Here's how the part is built. I have some questions about the finished solid (model axes, mm). Face numbers are marked on the shaded views. A direction names the side the tool comes from. Coordinates: 2 decimals unless noted, no trailing zeros. Write each loop counter-clockwise with the first axis right and the second up, starting at its lowest first coordinate (ties: lowest second). Pieces come first, ordered by that corner, then holes.
from build123d import *

# Parameters (mm, degrees)
F0_W     = 54
F0_H     = 150
F1_DEPTH = 50
F2_R     = 15
F3_R     = 15
F5_DEPTH = 5
F6_W     = 121.107407
F6_H     = 220.926333
F7_DEPTH = 5.001
F8_W     = 141.400545
F8_H     = 89.871116
F9_DEPTH = 50.001
F10_T    = -2.5


with BuildPart() as f1:
    # F0 (on Top) → F1 (new body)
    with BuildSketch(Plane.XY):
        Rectangle(F0_W, F0_H)
    extrude(amount=F1_DEPTH)

    # F2
    f2_edges = [f1.edges().sort_by_distance(p)[0] for p in [
        (27, -75, 25),
        (-27, -75, 25),
        (27, 75, 25),
        (-27, 75, 25),
    ]]
    fillet(f2_edges, radius=F2_R)

    # F3
    f3_edges = [f1.edges().sort_by_distance(p)[0] for p in [
        (-27, 0, 50),
    ]]
    fillet(f3_edges, radius=F3_R)

    # F4 (on face) → F5 (join)
    with BuildSketch(Plane(origin=(0, 0, 0), x_dir=(1, 0, 0), z_dir=(0, 0, -1))):
        with BuildLine():
            ThreePointArc((12, -75), (22.606602, -70.606602), (27, -60))
            Line((27, -60), (27, 60))
            ThreePointArc((27, 60), (22.606602, 70.606602), (12, 75))
            Line((12, 75), (-12, 75))
            ThreePointArc((-12, 75), (-22.606602, 70.606602), (-27, 60))
            Line((-27, 60), (-27, -60))
            ThreePointArc((-27, -60), (-22.606602, -70.606602), (-12, -75))
            Line((-12, -75), (12, -75))
        make_face()
    extrude(amount=F5_DEPTH)

    # F6 (on Top) → F7 (cut, through all)
    with BuildSketch(Plane.XY):
        with Locations((-1.455303, 11.194787)):
            Rectangle(F6_W, F6_H)
    extrude(amount=-F7_DEPTH, mode=Mode.SUBTRACT)

    # F8 (on face) → F9 (cut, through all)
    with BuildSketch(Plane(origin=(0, 0, 0), x_dir=(1, 0, 0), z_dir=(0, 0, -1))):
        with Locations((8.066163, -104.935558)):
            Rectangle(F8_W, F8_H)
    extrude(amount=-F9_DEPTH, mode=Mode.SUBTRACT)

    # F10
    f10_openings = [f1.faces().sort_by_distance(p)[0] for p in [
        (0, -6.638802, 0),
        (0, 60, 24.196941),
    ]]
    offset(amount=F10_T, openings=f10_openings)


solid = f1.part
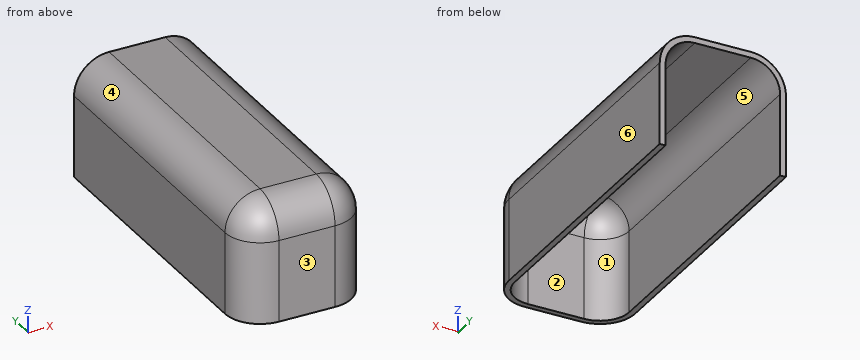
1. Thinking about a two-plate mould opening in X: for the marked faces 1, 2, 3 and 4, which applies, pulls with the +X half, pulls with the -X half, needs draft (parallel to the pull), parting line crosses it, or undercut?
2. On a 3-axis mill with a long thin cutter (end or side, diameter ignored), from which of +Z, -Z, +X, -X, +Y, -Y can I reach the whole of each face in a straight line? I mean the marked faces 5 and 6. Say none if no direction works.
3. I want a section at A-A (x = -3.5). List the corners of the cut face in (y, z) for me.
4. I want a section at B-B (z = 29.5). List the corners of the cut face in (x, y) for me.
5. I want a section at D-D (x = 20). List the corners of the cut face in (y, z) for me.
6. I want a section at C-C (y = -28.5). List the corners of the cut face in (x, z) for me, then the cut area to 3 significant figures.
7. If I drill on line 1 (X direction, y = -10, z = 17); line 2 (Y direction, x = -10, z = 33.5); line 3 (Z direction, x = 12.5, y = -32), over which ranges is the centre line in solid material (lowest first)?
8. For pin 1 Ø19 at (x, z) = (4.5, 19.5) entering from +Y; pin 2 Ø1 at (x, z) = (-17, 17.5) entering from -Y; pin 3 Ø2 at (x, y) = (-0.5, 41.5) entering from -Z, each with a flat end and sliding along its axis, tell me the tip position at first contact or that it passes through.
Response values:
1. face 1: undercut
1. face 2: undercut
1. face 3: needs draft
1. face 4: pulls with the -X half
2. face 5: -Z, +Y
2. face 6: +Z, -Z, +X, +Y, -Y
3. outline: (-75, 0) - (-72.5, 0) - (-72.5, 35) arc R12.5 cw to (-60, 47.5) - (60, 47.5) - (60, 50) - (-60, 50) arc R15 ccw to (-75, 35) - close
4. outline: (-27, -60) arc R15 ccw to (-12, -75) - (12, -75) arc R15 ccw to (27, -60) - (27, 60) - (24.5, 60) - (24.5, -60) arc R12.5 cw to (12, -72.5) - (-12, -72.5) arc R12.5 cw to (-24.5, -60) - (-24.5, 60) - (-27, 60) - close
5. outline: (-72.69, 0) - (-69.6, 0) - (-69.6, 35) arc R9.6 cw to (-60, 44.6) - (60, 44.6) - (60, 47.69) - (-60, 47.69) arc R12.69 ccw to (-72.69, 35) - close
6. outline: (-27, 0) - (-24.5, 0) - (-24.5, 35) arc R12.5 cw to (-12, 47.5) - (12, 47.5) arc R12.5 cw to (24.5, 35) - (24.5, 0) - (27, 0) - (27, 35) arc R15 ccw to (12, 50) - (-12, 50) arc R15 ccw to (-27, 35) - close
6. area: 343 mm2
7. line 1: x = -27 to -24.5, 24.5 to 27
7. line 2: y = -75 to -72.5
7. line 3: z = 47.49 to 49.99
8. pin 1: stops at y = -72.34
8. pin 2: stops at y = -74.31
8. pin 3: stops at z = 47.5
